Source: CAD feature listing. Evaluate the final solid. Frame: model axes, mm. Give positions to 0.01 mm unless a question says otherwise; leave off trailing zeros. Loops run counter-clockwise (first coordinate to the right, second up) from the corner with the lowest first, then second, coordinate; pieces in that order, holes last. Notation, with made-up numbers: M 86,-14 L 123,-14 A24 ccw 123,21 Z; hole C -15.75,24.25 d9. An arc over 180 degrees is marked long. Answer in a Markdown table with one row per item.
```python
from build123d import *

# Parameters (mm, degrees)
BOSS_EXTRUDE1_DEPTH = 6.35


with BuildPart() as part:
    # Sketch1 → Boss-Extrude1 (new body)
    with BuildSketch(Plane.XY):
        with BuildLine():
            Line((4.79079833, -60.96), (390.725573839, -60.96))
            ThreePointArc((390.725573839, -60.96), (543.389927897, 2.275645942), (606.625573839, 154.94))
            add(Edge.make_bspline(
                [(606.625573839, 154.94), (606.625573839, 316.01001421), (681.985382087, 368.523685091), (821.560436263, 399.924928327)],
                knots=[0, 0, 0, 0, 1, 1, 1, 1], degree=3))
            Line((821.560436263, 399.924928327), (821.560436263, 424.863249898))
            Line((821.560436263, 424.863249898), (702.170074113, 424.863249898))
            ThreePointArc((702.170074113, 424.863249898), (630.985008591, 399.990183462), (590.781410505, 336.196346076))
            ThreePointArc((590.781410505, 336.196346076), (456.769416888, 123.550221456), (219.485865145, 40.64))
            Line((219.485865145, 40.64), (4.79079833, 40.64))
            ThreePointArc((4.79079833, 40.64), (-13.169713912, 33.200512242), (-20.60920167, 15.24))
            Line((-20.60920167, 15.24), (-20.60920167, -35.56))
            ThreePointArc((-20.60920167, -35.56), (-13.169713912, -53.520512242), (4.79079833, -60.96))
        make_face()
    extrude(amount=BOSS_EXTRUDE1_DEPTH)


solid = part.part
```
Q1. Section query B-B (y = -12). Output: boundary loops of the cut face in (x, z), plus the area to 3 significant figures.
Values follow:
| item | result |
|---|---|
| outline | M -20.61,0 L 527.63,0 L 527.63,6.35 L -20.61,6.35 Z |
| area | 3,480 mm^2 |
Q2. Ray query, probe 1 along Y at (x, z) = (104, 3.5); probe 2 along X at (y, z) = (336.5, 4.75); probe 3 along X at (y, z) = (214.5, 3.75). Return the intervals inside material, ascending. Write a range as from..to.
Values follow:
| item | result |
|---|---|
| probe 1 | -60.96..40.64 |
| probe 2 | 590.85..672.88 |
| probe 3 | 539.26..610.73 |
Q3. Contact query for flat-ended pins moving along their axis: pin 1 Ø1.9 at (x, z) = (153.5, 4) entering from +Y; pin 2 Ø1 at (x, z) = (356.5, 3.5) entering from +Y; pin 3 Ø1 at (y, z) = (271.5, 2) entering from +X. Output: stop coordinate, or through.
Values follow:
| item | result |
|---|---|
| pin 1 | y = 40.64 |
| pin 2 | y = 66.32 |
| pin 3 | x = 626.27 |
Q4. Section query A-A (x = 95). Output: boundary loops of the cut face in (y, z), plus the area to 3 significant figures.
Values follow:
| item | result |
|---|---|
| outline | M -60.96,0 L 40.64,0 L 40.64,6.35 L -60.96,6.35 Z |
| area | 645 mm^2 |
